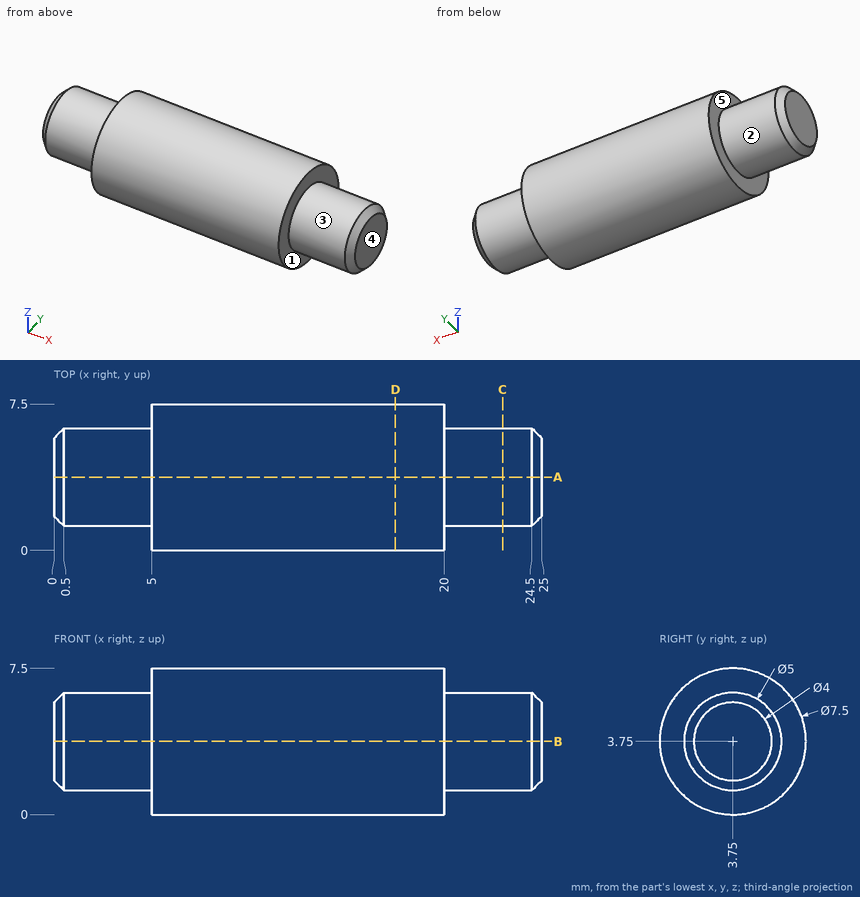
Here's the drawing with two shaded views (mm, measured from the low corner). I have some questions. A direction names the side the tool comes from. Give positions to 0.01 mm unless a question says otherwise; leave off trailing zeros. Order: outer loops, then holes, each group sorted by start corner. A loop starts at its lowest first (then second) coordinate and runs counter-clockwise, first axis right, second up. Notation, with made-up numbers: (77, 71) - (113, 71) arc R11 ccw to (113, 76) - close; hole circle Ø2 at (-16.5, -37.75). An arc over 180 degrees is marked (long way). Write each question's results on one line, items separated by ' | '.
1) Please list where these lines run through material, in increasing order: line 1 along X through (y, z) = (6.5, 2); line 2 along Z through (x, y) = (18.5, 0.5); line 3 along Y through (x, z) = (12.5, 2.5). Write a range as [from, to].
Final values:
line 1: x = [5, 20] | line 2: z = [1.88, 5.62] | line 3: y = [0.21, 7.29]
2) On a 3-axis mill with a long thin cutter (end or side, diameter ignored), from which of +Z, -Z, +X, -X, +Y, -Y can I reach the whole of each face in a straight line? I mean the marked faces 3, 4 and 5. Say none if no direction works.
Final values:
face 3: +X | face 4: +Z, -Z, +X, +Y, -Y | face 5: -X
3) Suppose I cut it at C-C, the plane x = 23. Write out the boundary of the cut face in (y, z), then the cut area to 3 significant figures.
Final values:
outline: circle Ø5 at (3.75, 3.75) | area: 19.6 mm^2
4) Suppose I cut it at D-D, the plane x = 17.5. Write out the boundary of the cut face in (y, z), then the cut area to 3 significant figures.
Final values:
outline: circle Ø7.5 at (3.75, 3.75) | area: 44.2 mm^2
5) Suppose I cut it at A-A, the plane y = 3.75. Write out the boundary of the cut face in (x, z), then the cut area to 3 significant figures.
Final values:
outline: (0, 1.75) - (0.5, 1.25) - (5, 1.25) - (5, 0) - (20, 0) - (20, 1.25) - (24.5, 1.25) - (25, 1.75) - (25, 5.75) - (24.5, 6.25) - (20, 6.25) - (20, 7.5) - (5, 7.5) - (5, 6.25) - (0.5, 6.25) - (0, 5.75) - close | area: 162 mm^2
6) If we mould it in two halves opening along Z, with no side actions, what happens to the marked faces 1 and 2? For each: pulls with the +Z half, pulls with the -Z half, needs draft (parallel to the pull), parting line crosses it, or undercut.
Final values:
face 1: needs draft | face 2: parting line crosses it
7) I'm going to push a flat-ended pin straight in: pin 1 Ø2 at (x, z) = (20.5, 3.5) entering from +Y. Where does the tip first touch, or does it pass through?
Final values:
pin 1: stops at y = 7.5
